Geometry check sheet. Reference: the model listing, model coordinates, mm. Round coordinates to 2 decimals unless told otherwise and drop trailing zeros. Write each loop counter-clockwise with the first axis right and the second up, starting at its lowest first coordinate (ties: lowest second). Pieces come first, ordered by that corner, then holes.
Item 1: Depth check by flat-ended pin: P1, Ø10, axis at x = -25.4, y = 25.4, coming from the -Z side. Enter the tip coordinate at first touch or a pass-through.
Item 2: Cross-section at B-B (x = -25.4). Enter the section's corners in (y, z), then the cut area to 3 significant figures.
Item 3: Draft check along Y on faces 1 (the face through (-4, 15, 6.35)), 2 (the face through (19.343, -78.107, 3.219)). Enter one of: pulls with the +Y half, pulls with the -Y half, needs draft (parallel to the pull), parting line crosses it, or undercut.
Item 4: Cross-section at A-A (y = -76.2). Enter the section's corners in (x, z).
Item 5: Scan line: probe 1 along Y at (x, z) = (25.4, 4.75). Record every from-to range of solid material in increasing order.
from build123d import *

# Parameters (mm, degrees)
SKETCH1_W           = 254
SKETCH1_H           = 152.4
SKETCH1_R           = 53.34
BOSS_EXTRUDE1_DEPTH = 6.35
BOSS_EXTRUDE2_START = -6.35
SKETCH13_R          = 53.34
BOSS_EXTRUDE2_DEPTH = 6.35
SKETCH21_W          = 431.8
SKETCH21_H          = 279.4
SKETCH21_W_2        = 254
SKETCH21_H_2        = 152.4
BOSS_EXTRUDE5_DEPTH = 6.35
SKETCH19_R          = 6.35
CUT_EXTRUDE5_DEPTH  = 265.346160366
SKETCH25_W          = 533.4
SKETCH25_H          = 330.2
SKETCH25_W_2        = 431.8
SKETCH25_H_2        = 279.4
BOSS_EXTRUDE7_DEPTH = 6.35


with BuildPart() as part:
    # Sketch1 → Boss-Extrude1 (new body)
    with BuildSketch(Plane.XY):
        Rectangle(SKETCH1_W, SKETCH1_H)
        Circle(SKETCH1_R, mode=Mode.SUBTRACT)
    extrude(amount=BOSS_EXTRUDE1_DEPTH)

    # Sketch13 → Boss-Extrude2 (add)
    with BuildSketch(Plane.XY.offset(6.35).offset(BOSS_EXTRUDE2_START)):
        Circle(SKETCH13_R)
    extrude(amount=BOSS_EXTRUDE2_DEPTH)

    # Sketch21 → Boss-Extrude5 (add)
    with BuildSketch(Plane.XY.offset(6.35)):
        with Locations((0, 12.7)):
            Rectangle(SKETCH21_W, SKETCH21_H)
        Rectangle(SKETCH21_W_2, SKETCH21_H_2, mode=Mode.SUBTRACT)
    extrude(amount=-BOSS_EXTRUDE5_DEPTH)

    # Sketch19 → Cut-Extrude5 (cut, through all)
    with BuildSketch(Plane.XY.offset(6.35)):
        with Locations((-25.4, 127)):
            Circle(SKETCH19_R)
        with Locations((-25.4, 25.4)):
            Circle(SKETCH19_R)
        with Locations(Location((25.4, 25.4, 0), (0, 0, 180))):
            Circle(SKETCH19_R)
        with Locations(Location((25.4, 127, 0), (0, 0, 180))):
            Circle(SKETCH19_R)
        with Locations((-25.4, -76.2)):
            Circle(SKETCH19_R)
        with Locations(Location((25.4, -76.2, 0), (0, 0, 180))):
            Circle(SKETCH19_R)
    extrude(amount=-CUT_EXTRUDE5_DEPTH, mode=Mode.SUBTRACT)

    # Sketch25 → Boss-Extrude7 (add)
    with BuildSketch(Plane.XY.offset(6.35)):
        with Locations((0, 12.7)):
            Rectangle(SKETCH25_W, SKETCH25_H)
        with Locations((0, 12.7)):
            Rectangle(SKETCH25_W_2, SKETCH25_H_2, mode=Mode.SUBTRACT)
    extrude(amount=-BOSS_EXTRUDE7_DEPTH)


solid = part.part
Resolved:
1. P1: passes through
2. outline: (-152.4, 0) - (-82.55, 0) - (-82.55, 6.35) - (-152.4, 6.35) - close; (-69.85, 0) - (19.05, 0) - (19.05, 6.35) - (-69.85, 6.35) - close; (31.75, 0) - (120.65, 0) - (120.65, 6.35) - (31.75, 6.35) - close; (133.35, 0) - (177.8, 0) - (177.8, 6.35) - (133.35, 6.35) - close
2. area: 1,850 mm2
3. face 1: needs draft
3. face 2: undercut
4. outline: (-266.7, 0) - (-31.75, 0) - (-31.75, 6.35) - (-266.7, 6.35) - close; (-19.05, 0) - (19.05, 0) - (19.05, 6.35) - (-19.05, 6.35) - close; (31.75, 0) - (266.7, 0) - (266.7, 6.35) - (31.75, 6.35) - close
5. probe 1: y = -152.4 to -82.55, -69.85 to 19.05, 31.75 to 120.65, 133.35 to 177.8
